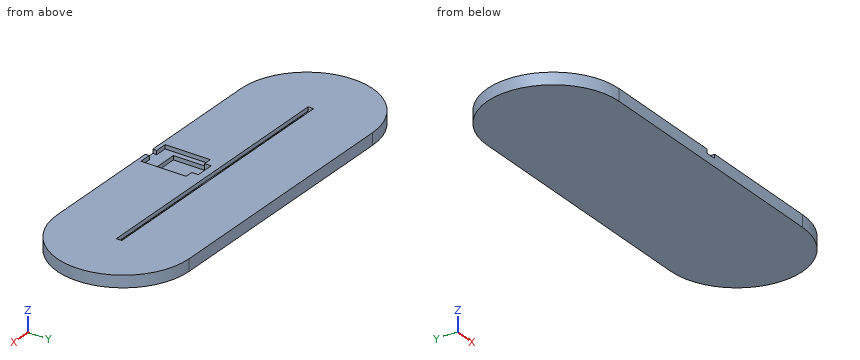
from build123d import *

# Parameters (mm, degrees)
PAD_DEPTH       = 3
PAD001_DEPTH    = 3
SKETCH002_W     = 209.08447
SKETCH002_H     = 4.18
PAD002_DEPTH    = 3
SKETCH003_W     = 26.3
SKETCH003_H     = 34.2
POCKET_DEPTH    = 3
SKETCH004_W     = 18
SKETCH004_H     = 25
POCKET001_DEPTH = 3
SKETCH005_W     = 14
SKETCH005_H     = 5
POCKET002_DEPTH = 6
SKETCH006_W     = 14
SKETCH006_H     = 3
POCKET003_DEPTH = 3
SKETCH007_W     = 8
SKETCH007_H     = 3
POCKET004_DEPTH = 3


with BuildPart() as part:
    # Sketch → Pad (new body)
    with BuildSketch(Plane.XY):
        with BuildLine():
            ThreePointArc((-100, 50), (-150, 0), (-100, -50))
            Line((-100, -50), (100, -50))
            ThreePointArc((100, -50), (150, 0), (100, 50))
            Line((-100, 50), (100, 50))
        make_face()
    extrude(amount=PAD_DEPTH)

    # Sketch001 (on Face6 of Pad) → Pad001 (join)
    with BuildSketch(Plane.XY.offset(3)):
        with BuildLine():
            ThreePointArc((-100, 50), (-150, 0), (-100, -50))
            Line((-100, -50), (100, -50))
            ThreePointArc((100, -50), (150, 0), (100, 50))
            Line((-100, 50), (100, 50))
        make_face()
        with BuildLine():
            ThreePointArc((-100, 5), (-105, 0), (-100, -5))
            Line((-100, -5), (100, -5))
            ThreePointArc((100, -5), (105, 0), (100, 5))
            Line((-100, 5), (100, 5))
        make_face(mode=Mode.SUBTRACT)
    extrude(amount=PAD001_DEPTH)

    # Sketch002 (on Face9 of Pad001) → Pad002 (join)
    with BuildSketch(Plane.XY.offset(6)):
        with BuildLine():
            ThreePointArc((-100, 50), (-150, 0), (-100, -50))
            Line((-100, -50), (100, -50))
            ThreePointArc((100, -50), (150, 0), (100, 50))
            Line((-100, 50), (100, 50))
        make_face()
        Rectangle(SKETCH002_W, SKETCH002_H, mode=Mode.SUBTRACT)
    extrude(amount=PAD002_DEPTH)

    # Sketch003 (on Face13 of Pad002) → Pocket (cut)
    with BuildSketch(Plane.XY.offset(9)):
        with Locations((0, -29.9)):
            Rectangle(SKETCH003_W, SKETCH003_H)
    extrude(amount=-POCKET_DEPTH, mode=Mode.SUBTRACT)

    # Sketch004 (on Face27 of Pocket) → Pocket001 (cut)
    with BuildSketch(Plane.XY.offset(6)):
        with Locations((0, -25.3)):
            Rectangle(SKETCH004_W, SKETCH004_H)
    extrude(amount=-POCKET001_DEPTH, mode=Mode.SUBTRACT)

    # Sketch005 (on Face13 of Pocket001) → Pocket002 (cut)
    with BuildSketch(Plane.XY.offset(9)):
        with Locations((0, -10.3)):
            Rectangle(SKETCH005_W, SKETCH005_H)
    extrude(amount=-POCKET002_DEPTH, mode=Mode.SUBTRACT)

    # Sketch006 (on Face23 of Pocket002) → Pocket003 (cut)
    with BuildSketch(Plane.XZ.offset(7.8)):
        with Locations((0, 4.5)):
            Rectangle(SKETCH006_W, SKETCH006_H)
    extrude(amount=-POCKET003_DEPTH, mode=Mode.SUBTRACT)

    # Sketch007 (on Face13 of Pocket003) → Pocket004 (cut)
    with BuildSketch(Plane.XY.offset(9)):
        with Locations((0, -48.5)):
            Rectangle(SKETCH007_W, SKETCH007_H)
    extrude(amount=-POCKET004_DEPTH, mode=Mode.SUBTRACT)


solid = part.part
Build history of the part. All positions in model axes, mm. Round coordinates to 2 decimals unless told otherwise and drop trailing zeros. Write each loop counter-clockwise with the first axis right and the second up, starting at its lowest first coordinate (ties: lowest second). Pieces come first, ordered by that corner, then holes. Notation, with made-up numbers: M -13.5,-10 L -4.5,-10 A21 ccw -4.5,3 Z; hole C -38.75,17 d1. An arc over 180 degrees is marked long. Use CSV: the item, a comma, the result in double quotes.
1. Saw through at D-D (x = 113.5). Give the cut face in (y, z), plus the area to 3 significant figures.
Reply:
outline,"M -48.14,0 L 48.14,0 L 48.14,9 L -48.14,9 Z"
area,"867 mm²"
2. Flat gauge pins, fed straight in: pin 1 (3.5 mm diameter, centred on y = -27, z = 7, fed in from +X); pin 2 (13 mm diameter, centred on x = -2.5, y = -40, fed in from +Z); pin 3 (1.5 mm diameter, centred on y = 37.5, z = 3, fed in from -X); pin 4 (10 mm diameter, centred on x = 17, y = -18, fed in from -Z). Where does each tip first touch, or does it go through?
Reply:
pin 1,"stops at x = 143.16"
pin 2,"stops at z = 6"
pin 3,"stops at x = -133.9"
pin 4,"stops at z = 0"
3. Saw through at A-A (z = 7.5). Give the cut face in (x, y), plus the area to 3 significant figures.
Reply:
outline,"M -100,-50 L -4,-50 L -4,-47 L -13.15,-47 L -13.15,-12.8 L -7,-12.8 L -7,-7.8 L 7,-7.8 L 7,-12.8 L 13.15,-12.8 L 13.15,-47 L 4,-47 L 4,-50 L 100,-50 A50 ccw 100,50 L -100,50 A50 ccw Z; hole M -104.54,-2.09 L 104.54,-2.09 L 104.54,2.09 L -104.54,2.09 Z"
area,"26,000 mm²"
4. Saw through at B-B (x = 0). Give the cut face in (y, z).
Reply:
outline,"M -50,0 L 50,0 L 50,9 L 2.09,9 L 2.09,6 L 5,6 L 5,3 L -37.8,3 L -37.8,6 L -50,6 Z; M -7.8,6 L -2.09,6 L -2.09,9 L -7.8,9 Z"
5. Wall check: probe 1 along Y at (x, z) = (-87.5, 3.5); probe 2 along X at (y, z) = (-35.5, 7.75); probe 3 along X at (y, z) = (-4, 5). Give the ranges that are in metal, low to high. Write a range as from..to.
Reply:
probe 1,"y = -50..-5, 5..50"
probe 2,"x = -135.21..-13.15, 13.15..135.21"
probe 3,"x = -149.84..-103, 103..149.84"
6. Saw through at C-C (x = 58). Give the cut face in (y, z).
Reply:
outline,"M -50,0 L 50,0 L 50,9 L 2.09,9 L 2.09,6 L 5,6 L 5,3 L -5,3 L -5,6 L -2.09,6 L -2.09,9 L -50,9 Z"
